Verification items for the finished model (mm, model axes). Face numbers are marked on the shaded views. A direction names the side the tool comes from. Round coordinates to 2 decimals unless told otherwise and drop trailing zeros. Order: outer loops, then holes, each group sorted by start corner. A loop starts at its lowest first (then second) coordinate and runs counter-clockwise, first axis right, second up. Notation, with made-up numbers: (79, 69) -> (116, 69) arc R10 cw to (116, 83) -> close; hole circle Ø9 at (21.25, 79). An arc over 180 degrees is marked (long way). Put each result on its own line as item: value.
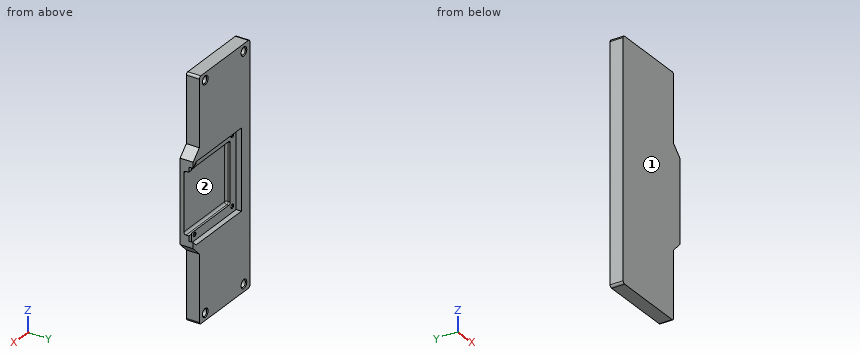
```python
from build123d import *

# Parameters (mm, degrees)
BOSS_EXTRUDE1_DEPTH     = 11.5
SKETCH4_R               = 3.075
CUT_EXTRUDE1_DEPTH      = 6
BOSS_EXTRUDE3_DEPTH     = 11.5
CUT_EXTRUDE6_DEPTH      = 4.6
CUT_EXTRUDE3_DEPTH      = 114.485065097
CUT_EXTRUDE3_DEPTH_BACK = 3.7
SKETCH24_W              = 57
SKETCH24_H              = 54
SKETCH25_R              = 1.35
CUT_EXTRUDE4_DEPTH      = 5
CHAMFER4_SIZE           = 0.5
FILLET1_R               = 2
BOSS_EXTRUDE2_DEPTH     = 0.8
CHAMFER5_SIZE           = 0.75


with BuildPart() as part:
    # Sketch1 → Boss-Extrude1 (new body)
    with BuildSketch(Plane(origin=(0, 0, 0), x_dir=(1, 0, 0), z_dir=(0, 1, 0))):
        with BuildLine():
            Line((-34.125, 90), (-34.125, -90))
            Line((-34.125, -90), (-34.125, -103))
            ThreePointArc((-34.125, -103), (-33.539213562, -104.414213562), (-32.125, -105))
            Line((-32.125, -105), (32.125, -105))
            ThreePointArc((32.125, -105), (33.539213562, -104.414213562), (34.125, -103))
            Line((34.125, -103), (34.125, -90))
            Line((34.125, -90), (34.125, 90))
            Line((34.125, 90), (34.125, 103))
            ThreePointArc((34.125, 103), (33.539213562, 104.414213562), (32.125, 105))
            Line((32.125, 105), (-32.125, 105))
            ThreePointArc((-32.125, 105), (-33.539213562, 104.414213562), (-34.125, 103))
            Line((-34.125, 103), (-34.125, 90))
        make_face()
    extrude(amount=BOSS_EXTRUDE1_DEPTH)

    # Sketch4 → Cut-Extrude1 (cut)
    with BuildSketch(Plane(origin=(0, 11.5, 0), x_dir=(1, 0, 0), z_dir=(0, 1, 0))):
        with Locations(Location((-26.125, -98.5, 0), (0, 0, 270))):
            Circle(SKETCH4_R)
        with Locations(Location((26.125, -98.5, 0), (0, 0, 270))):
            Circle(SKETCH4_R)
        with Locations(Location((26.125, 98.5, 0), (0, 0, 270))):
            Circle(SKETCH4_R)
        with Locations(Location((-26.125, 98.5, 0), (0, 0, 270))):
            Circle(SKETCH4_R)
    extrude(amount=-CUT_EXTRUDE1_DEPTH, mode=Mode.SUBTRACT)

    # Sketch27 → Boss-Extrude3 (add)
    with BuildSketch(Plane(origin=(0, 11.5, 0), x_dir=(1, 0, 0), z_dir=(0, 1, 0))):
        Polygon((34.125, 45), (42.5, 36.625), (42.5, -36.625), (34.125, -45), align=None)
    extrude(amount=-BOSS_EXTRUDE3_DEPTH)

    # Sketch21 → Cut-Extrude6 (cut)
    with BuildSketch(Plane(origin=(0, 11.5, 0), x_dir=(1, 0, 0), z_dir=(0, 1, 0))):
        Polygon((42.5, 31.353553391), (42.5, -31.353553391), (38.603553391, -35.25), (-22.75, -35.25), (-22.75, 35.25), (38.603553391, 35.25), align=None)
    extrude(amount=-CUT_EXTRUDE6_DEPTH, mode=Mode.SUBTRACT)

    # Sketch24 → Cut-Extrude3 (cut, two sides: drawn at the far end of the back side and taken through both)
    with BuildSketch(Plane(origin=(0, 6.9, 0), x_dir=(1, 0, 0), z_dir=(0, 1, 0)).offset(-CUT_EXTRUDE3_DEPTH_BACK)):
        with Locations((14, 0)):
            Rectangle(SKETCH24_W, SKETCH24_H)
    extrude(amount=CUT_EXTRUDE3_DEPTH + CUT_EXTRUDE3_DEPTH_BACK, mode=Mode.SUBTRACT)

    # Sketch25 → Cut-Extrude4 (cut)
    with BuildSketch(Plane(origin=(0, 6.9, 0), x_dir=(1, 0, 0), z_dir=(0, 1, 0))):
        with Locations(Location((33.5, 30, 0), (0, 0, 270))):
            Circle(SKETCH25_R)
        with Locations(Location((-17.5, 30, 0), (0, 0, 270))):
            Circle(SKETCH25_R)
        with Locations(Location((33.5, -30, 0), (0, 0, 270))):
            Circle(SKETCH25_R)
        with Locations(Location((-17.5, -30, 0), (0, 0, 270))):
            Circle(SKETCH25_R)
    extrude(amount=-CUT_EXTRUDE4_DEPTH, mode=Mode.SUBTRACT)

    # Chamfer4
    chamfer4_edges = [part.edges().sort_by_distance(p)[0] for p in [
        (-17.5, 6.9, -31.35),
        (33.5, 6.9, 28.65),
        (-17.5, 6.9, 28.65),
        (33.5, 6.9, -31.35),
    ]]
    chamfer(chamfer4_edges, length=CHAMFER4_SIZE)

    # Fillet1
    fillet1_edges = [part.edges().sort_by_distance(p)[0] for p in [
        (14, 3.2, -27),
        (-14.5, 5.05, -27),
        (-14.5, 3.2, 0),
        (-14.5, 5.05, 27),
        (14, 3.2, 27),
    ]]
    fillet(fillet1_edges, radius=FILLET1_R)

    # Sketch26 → Boss-Extrude2 (add)
    with BuildSketch(Plane(origin=(0, 6.9, 0), x_dir=(1, 0, 0), z_dir=(0, 1, 0))):
        Polygon((38.603553391, 35.25), (38.603553391, 27), (42.5, 27), (42.5, 31.353553391), align=None)
        Polygon((42.5, -31.353553391), (38.603553391, -35.25), (38.603553391, -27), (42.5, -27), align=None)
    extrude(amount=BOSS_EXTRUDE2_DEPTH)

    # Chamfer5
    chamfer5_edges = [part.edges().sort_by_distance(p)[0] for p in [
        (-26.125, 11.5, -101.575),
        (26.125, 11.5, -101.575),
        (26.125, 11.5, 95.425),
        (-26.125, 11.5, 95.425),
    ]]
    chamfer(chamfer5_edges, length=CHAMFER5_SIZE)


solid = part.part
```
Item 1: Tool access check on the marked faces 1 and 2. Record the directions out of +Z, -Z, +X, -X, +Y, -Y that give a thin tool (end or side, any length) a straight path to the whole face; none if there is none.
Geometry check:
face 1: +Z, -Z, +X, -X, -Y
face 2: +X, +Y
Item 2: Depth check by flat-ended pin: pin 1 Ø4 at (x, z) = (9.5, -1) entering from +Y; pin 2 Ø1 at (y, z) = (4.5, -42) entering from +X (3 decimals); pin 3 Ø5 at (x, z) = (26, -99) entering from +Y; pin 4 Ø3.5 at (x, z) = (-17.5, -30) entering from -Y. Enter the tip coordinate at first touch or a pass-through.
Geometry check:
pin 1: y = 3.2
pin 2: x = 37.625
pin 3: y = 5.5
pin 4: y = 0
Item 3: Sectioned sample at C-C, the plane z = 9.5. Record the boundary of the cut face in (x, y) (3 decimals).
Geometry check:
outline: (-34.125, 0) -> (42.5, 0) -> (42.5, 3.2) -> (-12.5, 3.2) arc R2 cw to (-14.5, 5.2) -> (-14.5, 6.9) -> (-22.75, 6.9) -> (-22.75, 11.5) -> (-34.125, 11.5) -> close
Item 4: Sectioned sample at B-B, the plane x = -9. Record the boundary of the cut face in (y, z).
Geometry check:
outline: (0, -105) -> (11.5, -105) -> (11.5, -35.25) -> (6.9, -35.25) -> (6.9, -27) -> (5.2, -27) arc R2 cw to (3.2, -25) -> (3.2, 25) arc R2 cw to (5.2, 27) -> (6.9, 27) -> (6.9, 35.25) -> (11.5, 35.25) -> (11.5, 105) -> (0, 105) -> close
Item 5: Sectioned sample at A-A, the plane z = -98.5. Record the boundary of the cut face in (x, y) (3 decimals).
Geometry check:
outline: (-34.125, 0) -> (34.125, 0) -> (34.125, 11.5) -> (29.95, 11.5) -> (29.2, 10.75) -> (29.2, 5.5) -> (23.05, 5.5) -> (23.05, 10.75) -> (22.3, 11.5) -> (-22.3, 11.5) -> (-23.05, 10.75) -> (-23.05, 5.5) -> (-29.2, 5.5) -> (-29.2, 10.75) -> (-29.95, 11.5) -> (-34.125, 11.5) -> close
Item 6: Material ranges on line 1 along X through (y, z) = (4.4, 30) (3 decimals); line 2 along X through (y, z) = (7.2, 98.5) (3 decimals); line 3 along Z through (x, y) = (-22, 8), recorded low to high.
Geometry check:
line 1: -34.125 to -18.85, -16.15 to 32.15, 34.85 to 42.5
line 2: -34.125 to -29.2, -23.05 to 23.05, 29.2 to 34.125
line 3: -105 to -35.25, 35.25 to 105
Item 7: Sectioned sample at D-D, the plane z = 88. Record the boundary of the cut face in (x, y) (3 decimals).
Geometry check:
outline: (-34.125, 0) -> (34.125, 0) -> (34.125, 11.5) -> (-34.125, 11.5) -> close
